Autodesk Inventor part; units mm, degrees
ref_plane "YZ Plane" through (0, 0, 0) normal (1, 0, 0) x (0, 1, 0)
ref_plane "XZ Plane" through (0, 0, 0) normal (0, 1, 0) x (-1, 0, 0)
ref_plane "XY Plane" through (0, 0, 0) normal (0, 0, 1) x (1, 0, 0)
sketch "Sketch1" plane through (0, 0, 0) normal (0, 0, 1) x (1, 0, 0)
  line L0 (0, 0) -> (0, -38.8)
  line L1 (0, 0) -> (7, 0)
  line L2 (9, -2) -> (9, -2)
  line L3 (8.5, -2.5) -> (3.5, -2.5)
  line L4 (3.5, -2.5) -> (3.5, -18.5)
  line L5 (3.5, -18.5) -> (4, -18.5)
  line L6 (4, -18.5) -> (4, -33.5)
  line L7 (4, -33.5) -> (3.125, -33.5)
  line L8 (3.125, -33.5) -> (3.125, -38.8)
  line L9 (3.125, -38.8) -> (2.4322, -40)
  line L10 (2.4322, -40) -> (1.2738, -40)
  arc A0 (8.5, -2.5) -> (9, -2) centre (8.5, -2) ccw
  arc A1 (9, -2) -> (7, 0) centre (7, -2) ccw
  line L11 (0, -38.8) -> (1.2738, -40)
  dimension "d1" = 2.5
  dimension "d2" = 16
  dimension "d3" = 15
  dimension "d4" = 1.2
  dimension "d5" = 60
  dimension "d6" = 3.125
  dimension "d7" = 3.5
  dimension "d8" = 4
  dimension "d9" = 9
  dimension "d10" = 0.5
  dimension "d11" = 2
  dimension "d12" = 1.75
  dimension "d15" = 40
revolve "Revolution1" add sketch "Sketch1" angle 360 about axis through (0, 0, 0) along (0, -1, 0)
fillet "Fillet1" radius 0.1 2 edges at (-3.125, -33.5, 0) (-3.5, -18.5, 0)
fillet "Fillet2" radius 0.25 1 edges at (-3.5, -2.5, 0)
properties part number "100-02" material "Stainless Steel"
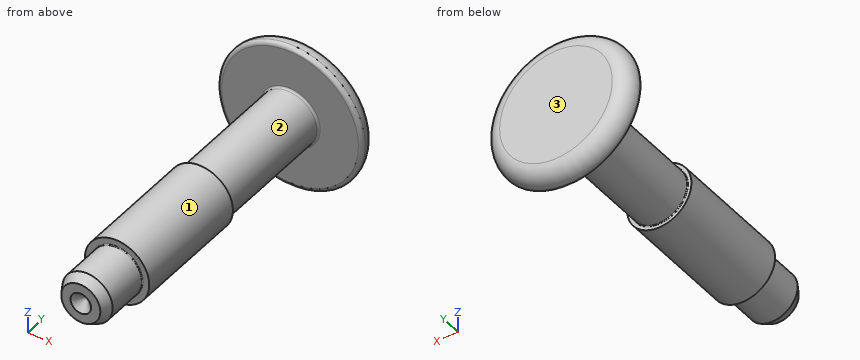
Could you check a few things on this model? Use its own coordinates, in mm. Face numbers are marked on the shaded views. Round coordinates to 2 decimals unless told otherwise and drop trailing zeros. Loops run counter-clockwise (first coordinate to the right, second up) from the corner with the lowest first, then second, coordinate; pieces in that order, holes last. Notation, with made-up numbers: (35, 15.25) - (82, 15.25) arc R10 ccw to (82, 26.25) - close; hole circle Ø2 at (19, -2). An arc over 180 degrees is marked (long way). Use CSV: the item, a comma, the result in double quotes.
Item 1: If we section it at B-B on y = -27: List the corners of the cut face in (x, z) for me.
Here are the results:
outline,"circle Ø8 at (0, 0)"
Item 2: I need wall thicknesses on L1, parallel to Y at x = 2.25, z = 3.25; L2, parallel to Z at x = -2.5, y = -27; L3, parallel to Y at x = 1.25, z = 3. Which ranges of each line are inside material? Lowest first, please. Write a range as [from, to].
Here are the results:
L1,"y = [-33.5, -18.5], [-2.5, 0]"
L2,"z = [-3.12, 3.12]"
L3,"y = [-33.5, 0]"
Item 3: Will these pins go through, and if not, where does the flat tip stop? pin 1 (4 mm diameter, centred on y = -21, z = 1.5, fed in from +X); pin 2 (1.5 mm diameter, centred on x = 0, z = -2.5, fed in from +Y); pin 3 (4 mm diameter, centred on y = -28, z = -5, fed in from -X); pin 4 (10 mm diameter, centred on y = -36, z = -4.5, fed in from -X).
Here are the results:
pin 1,"stops at x = 4"
pin 2,"stops at y = 0"
pin 3,"stops at x = -2.65"
pin 4,"stops at x = -4"
Item 4: If we mould it in two halves opening along Y, with no side actions, what happens to the marked faces 1, 2 and 3? For each: pulls with the +Y half, pulls with the -Y half, needs draft (parallel to the pull), parting line crosses it, or undercut.
Here are the results:
face 1,"needs draft"
face 2,"undercut"
face 3,"pulls with the +Y half"
Item 5: If we section it at A-A on y = -5: List the corners of the cut face in (x, z) for me.
Here are the results:
outline,"circle Ø7 at (0, 0)"
